Check sheet for the drawn part. Datum: minimum x, y, z corner. Units: mm. A direction names the side the tool comes from. Give positions to 0.01 mm unless a question says otherwise; leave off trailing zeros. Order: outer loops, then holes, each group sorted by start corner. A loop starts at its lowest first (then second) coordinate and runs counter-clockwise, first axis right, second up. Notation, with made-up numbers: M 88.25,57.5 L 142.25,57.5 A7 ccw 142.25,69.5 Z; hole C 83.5,44 d7. An arc over 180 degrees is marked long. Answer in a Markdown table with one row per item. Add a question column.
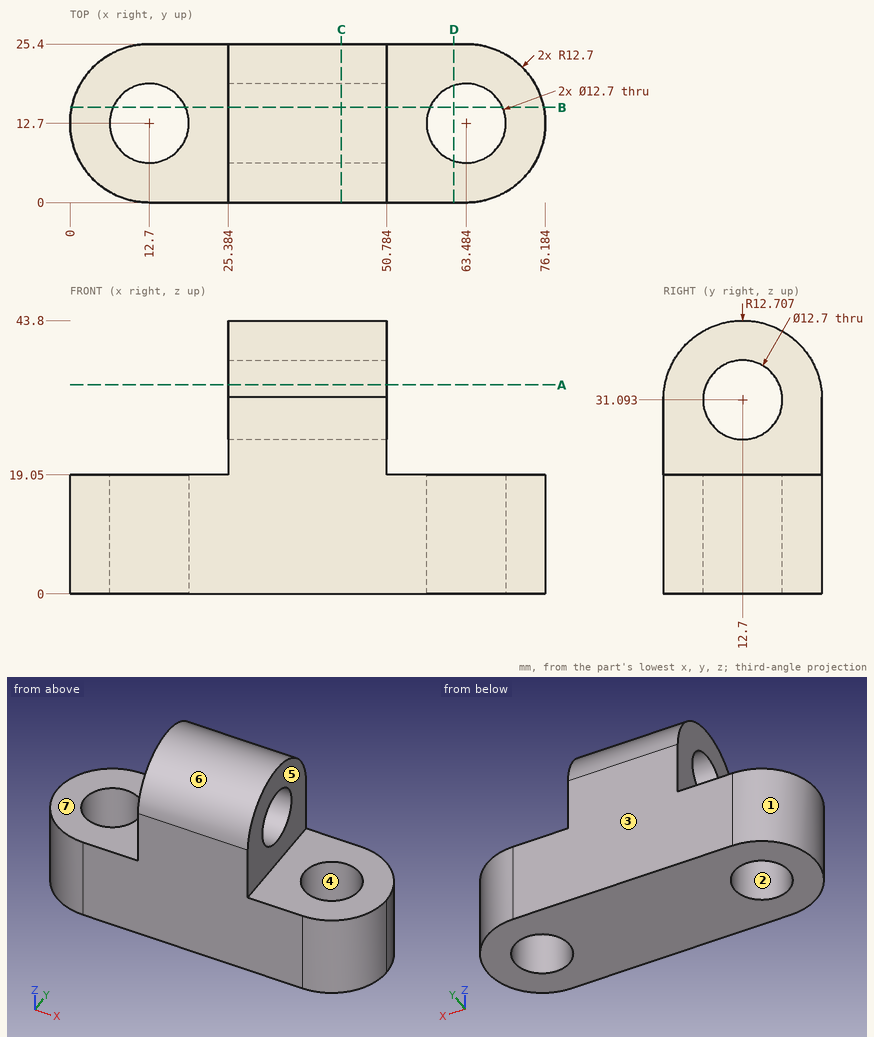
Q1. Thickness scan on probe 1 along X at (y, z) = (13, 9); probe 2 along Z at (x, y) = (33.25, 12.7); probe 3 along X at (y, z) = (18, 13) (1 decimal). Record the ranges inside material, lowest first.
Q2. Tool access check on the marked faces 5, 6 and 7. Record the directions out of +Z, -Z, +X, -X, +Y, -Y that give a thin tool (end or side, any length) a straight path to the whole face; none if there is none.
Q3. Cross-section at A-A (z = 33.5). Record the boundary of the cut face in (x, y).
Q4. Cross-section at D-D (x = 61.5). Record the boundary of the cut face in (y, z).
Q5. Cross-section at B-B (y = 15.25). State how many separate pieces and enclosed holes the cut face has, and give its area (4 significant figures).
Q6. Cross-section at C-C (x = 43.5). Record the boundary of the cut face in (y, z), and give its area (3 significant figures).
Q7. Go/stop test with flat-tipped pins: pin 1 (2 mm diameter, centred on y = 2.5, z = 19.5, fed in from -X); pin 2 (10 mm diameter, centred on y = 16, z = 32.5, fed in from +X); pin 3 (12.5 mm diameter, centred on y = 12, z = 27, fed in from -X); pin 4 (7.5 mm diameter, centred on y = 12.7, z = 31.09, fed in from +X). Record where each tip stops, or that it passes through.
Q8. Draft check along Y on the marked faces 1, 2, 3 and 4. Enter one of: pulls with the +Y half, pulls with the -Y half, needs draft (parallel to the pull), parting line crosses it, or undercut.
Values follow:
| question | item | result |
|---|---|---|
| 1 | probe 1 | 0 to 6.36, 19.04 to 57.14, 69.83 to 76.18 |
| 1 | probe 2 | 0 to 24.74, 37.44 to 43.8 |
| 1 | probe 3 | 1.2 to 9.2, 16.2 to 60, 67 to 75 |
| 2 | face 5 | +Z, +X, +Y, -Y |
| 2 | face 6 | +Z, +X, -X |
| 2 | face 7 | +Z, -X, +Y, -Y |
| 3 | outline | M 25.38,0.22 L 50.78,0.22 L 50.78,6.82 L 25.38,6.82 Z; M 25.38,18.58 L 50.78,18.58 L 50.78,25.18 L 25.38,25.18 Z |
| 4 | outline | M 0,0 L 6.67,0 L 6.67,19.05 L 0,19.05 Z; M 18.73,0 L 25.4,0 L 25.4,19.05 L 18.73,19.05 Z |
| 5 | separate pieces | 4 |
| 5 | enclosed holes | 0 |
| 5 | area | 1,325 mm² |
| 6 | outline | M 0,0 L 25.4,0 L 25.4,31.51 A12.71 ccw 0,31.51 Z; hole C 12.7,31.09 d12.7 |
| 6 | area | 917 mm² |
| 7 | pin 1 | x = 4.06 |
| 7 | pin 2 | x = 50.78 |
| 7 | pin 3 | x = 25.38 |
| 7 | pin 4 | through |
| 8 | face 1 | parting line crosses it |
| 8 | face 2 | undercut |
| 8 | face 3 | pulls with the +Y half |
| 8 | face 4 | undercut |
